The drawing under review shows one solid part. Ordinate dimensions are in mm from its lowest x, y, z. A direction names the side the tool comes from. Coordinates: 2 decimals unless noted, no trailing zeros. Order: outer loops, then holes, each group sorted by start corner. A loop starts at its lowest first (then second) coordinate and runs counter-clockwise, first axis right, second up.
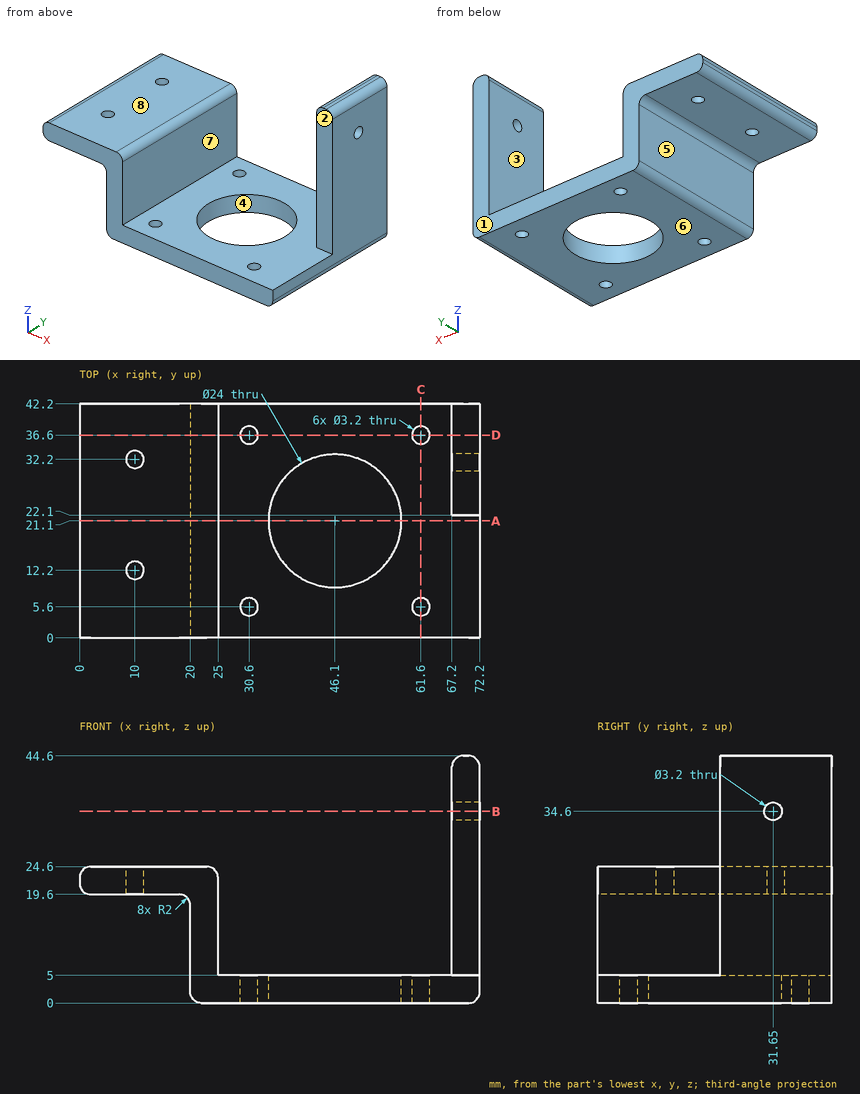
(1) Consider section B-B (z = 34.6). Give the boundary of the cut face in (x, y), then the cut area to 3 significant figures.
(2) Wall thickness on line 1 (Z direction, x = 69.2, y = 31.65); line 2 (X direction, y = 5.6, z = 2.05); line 3 (X direction, y = 12, z = 22): over which ranges is each line inside the solid? List them lowest first.
(3) Tool access review of the marked faces 5, 6, 7 and 8: name each direction out of +Z, -Z, +X, -X, +Y, -Y from which nothing blocks a thin tool from reaching the whole face with its end or side.
(4) Consider section A-A (y = 21.1). Give the boundary of the cut face in (x, z), then the cut area to 3 significant figures.
(5) The part is to be moulded in two halves that separate along Y. For the marked faces 1, 2, 3 and 4, say which applies: +Y half, -Y half, draft (parallel to the pull), parting line (faces both ways), or undercut.
(6) Insertion check: pin 1 Ø5.5 at (x, z) = (69, 22.5) entering from -Y; pin 2 Ø8 at (y, z) = (11.5, 14.5) entering from -X; pin 3 Ø3.5 at (x, y) = (10, 32.2) entering from -Z; pin 4 Ø3 at (x, y) = (61.6, 36.6) entering from +Z. Each pin has a flat end and moves straight along its axis. Give the tip position at first contact, or say it passes through.
(7) Consider section D-D (y = 36.6). Give the boundary of the cut face in (x, z), then the cut area to 3 significant figures.
(8) Consider section C-C (x = 61.6). Give the boundary of the cut face in (y, z), then the cut area to 3 significant figures.
Findings:
1. outline: (67.2, 22.1) - (72.2, 22.1) - (72.2, 30.05) - (67.2, 30.05) - close; (67.2, 33.25) - (72.2, 33.25) - (72.2, 42.2) - (67.2, 42.2) - close
1. area: 84.5 mm2
2. line 1: z = 0 to 33, 36.2 to 44.6
2. line 2: x = 20 to 29, 32.2 to 60, 63.2 to 72.2
2. line 3: x = 0 to 8.41, 11.59 to 25
3. face 5: -Z, -X, +Y, -Y
3. face 6: -Z, +X, -X, +Y, -Y
3. face 7: +Z, +Y, -Y
3. face 8: +Z, -X, +Y, -Y
4. outline: (0, 21.6) arc R2 ccw to (2, 19.6) - (18, 19.6) arc R2 cw to (20, 17.6) - (20, 2) arc R2 ccw to (22, 0) - (34.1, 0) - (34.1, 5) - (25, 5) - (25, 22.6) arc R2 ccw to (23, 24.6) - (2, 24.6) arc R2 ccw to (0, 22.6) - close; (58.1, 0) - (70.2, 0) arc R2 ccw to (72.2, 2) - (72.2, 5) - (58.1, 5) - close
4. area: 336 mm2
5. face 1: +Y half
5. face 2: -Y half
5. face 3: draft
5. face 4: undercut
6. pin 1: stops at y = 22.1
6. pin 2: stops at x = 19.79
6. pin 3: stops at z = 19.6
6. pin 4: passes through
7. outline: (0, 21.6) arc R2 ccw to (2, 19.6) - (18, 19.6) arc R2 cw to (20, 17.6) - (20, 2) arc R2 ccw to (22, 0) - (29, 0) - (29, 5) - (25, 5) - (25, 22.6) arc R2 ccw to (23, 24.6) - (2, 24.6) arc R2 ccw to (0, 22.6) - close; (32.2, 0) - (60, 0) - (60, 5) - (32.2, 5) - close; (63.2, 0) - (70.2, 0) arc R2 ccw to (72.2, 2) - (72.2, 42.6) arc R2 ccw to (70.2, 44.6) - (69.2, 44.6) arc R2 ccw to (67.2, 42.6) - (67.2, 5) - (63.2, 5) - close
7. area: 620 mm2
8. outline: (0, 0) - (4, 0) - (4, 5) - (0, 5) - close; (7.2, 0) - (35, 0) - (35, 5) - (7.2, 5) - close; (38.2, 0) - (42.2, 0) - (42.2, 5) - (38.2, 5) - close
8. area: 179 mm2
